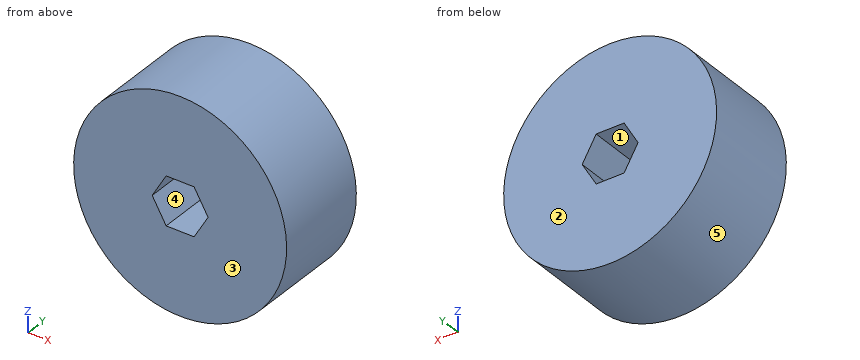
```python
from build123d import *

# Parameters (mm, degrees)
SKETCH1_R           = 27.94
BOSS_EXTRUDE1_DEPTH = 25.4
CUT_EXTRUDE1_DEPTH  = 47.972834703


with BuildPart() as part:
    # Sketch1 → Boss-Extrude1 (new body)
    with BuildSketch(Plane(origin=(0, 0, 0), x_dir=(1, 0, 0), z_dir=(0, 1, 0))):
        with Locations(Location((0, 0, 0), (0, 0, 270))):
            Circle(SKETCH1_R)
    extrude(amount=BOSS_EXTRUDE1_DEPTH)

    # Sketch2 → Cut-Extrude1 (cut, through all)
    with BuildSketch(Plane.XZ):
        Polygon((-3.666174209, 6.35), (-7.332348419, 0), (-3.666174209, -6.35), (3.666174209, -6.35), (7.332348419, 0), (3.666174209, 6.35), align=None)
    extrude(amount=-CUT_EXTRUDE1_DEPTH, mode=Mode.SUBTRACT)


solid = part.part
```
Input: part model. Units: mm. Frame: model coordinates. Face numbers are marked on the shaded views. A direction names the side the tool comes from. Give positions to 0.01 mm unless a question says otherwise; leave off trailing zeros. Order: outer loops, then holes, each group sorted by start corner. A loop starts at its lowest first (then second) coordinate and runs counter-clockwise, first axis right, second up. Notation, with made-up numbers: (84.25, 79) -> (113.25, 79) arc R34 cw to (113.25, 111) -> close; hole circle Ø5 at (-24, 50.25). An arc over 180 degrees is marked (long way). Write each question's results on one line, items separated by ' | '. Start each with the question number.
Item 1: Line query: line 1 (Z direction, x = -0.5, y = 17.25); line 2 (Z direction, x = 6.5, y = 3.25); line 3 (X direction, y = 11.5, z = 5). Output: solid intervals per line, ascending.
Item 2: Set-up query: the marked faces 1 and 2. Return all of +Z, -Z, +X, -X, +Y, -Y with unobstructed straight access to the full face (end or side cutting, diameter ignored); none if empty.
Item 3: Cut plane B-B on y = 11. Return the cut outline in (x, z), then the cut area to 3 significant figures.
Item 4: Mould query, pull axis X, two halves, no side actions, for the marked faces 3, 4 and 5. Classes: pulls with the +X half, pulls with the -X half, needs draft (parallel to the pull), parting line crosses it, or undercut.
Item 5: Cut plane A-A on x = 0. Return the cut outline in (y, z).
Item 6: Contact query for flat-ended pins moving along their axis: P1, Ø5, axis at x = 0.5, z = 3, coming from the +Y side; P2, Ø3, axis at x = -8, y = 3.5, coming from the +Z side; P3, Ø3, axis at y = 6.5, z = -11.5, coming from the +X side; P4, Ø1, axis at y = 12, z = -0.5, coming from the -X side. Output: stop coordinate, or through.
Item 7: Cut plane D-D on z = 8. Return the cut outline in (x, y), then the cut area to 3 significant figures.
Item 8: Cut plane C-C on z = -1. Return the cut outline in (x, y) (3 decimals).
Established:
1) line 1: -27.94 to -6.35, 6.35 to 27.94 | line 2: -27.17 to -1.44, 1.44 to 27.17 | line 3: -27.49 to -4.45, 4.45 to 27.49
2) face 1: +Y, -Y | face 2: +Z, -Z, +X, -X, +Y
3) outline: circle Ø55.88 at (0, 0); hole (-7.33, 0) -> (-3.67, -6.35) -> (3.67, -6.35) -> (7.33, 0) -> (3.67, 6.35) -> (-3.67, 6.35) -> close | area: 2,310 mm^2
4) face 3: needs draft | face 4: undercut | face 5: parting line crosses it
5) outline: (0, -27.94) -> (25.4, -27.94) -> (25.4, -6.35) -> (0, -6.35) -> close; (0, 6.35) -> (25.4, 6.35) -> (25.4, 27.94) -> (0, 27.94) -> close
6) P1: through | P2: z = 27.17 | P3: x = 26.09 | P4: x = -27.94
7) outline: (-26.77, 0) -> (26.77, 0) -> (26.77, 25.4) -> (-26.77, 25.4) -> close | area: 1,360 mm^2
8) outline: (-27.922, 0) -> (-6.755, 0) -> (-6.755, 25.4) -> (-27.922, 25.4) -> close; (6.755, 0) -> (27.922, 0) -> (27.922, 25.4) -> (6.755, 25.4) -> close
